```python
from build123d import *

# Parameters (mm, degrees)
BOSS_EXTRUDE1_DEPTH = 52.5
RIB1_REACH          = 184.705
SKETCH3_WALL_W      = 451.226000884
SKETCH3_WALL_H      = 25
RIB2_REACH          = 184.705
SKETCH2_WALL_W      = 451.226000884
SKETCH2_WALL_H      = 25
CUT_EXTRUDE1_DEPTH  = 31


with BuildPart() as part:
    # Sketch1 → Boss-Extrude1 (new, symmetric)
    with BuildSketch(Plane(origin=(0, 0, 0), x_dir=(0, 0, -1), z_dir=(1, 0, 0))):
        with BuildLine():
            Line((45, 0), (105, 0))
            Line((105, 0), (105, 60))
            Line((105, 60), (80, 60))
            Line((80, 60), (80, 140))
            Line((80, 140), (20, 140))
            Line((20, 140), (20, 126.52173913))
            Line((20, 126.52173913), (45, 126.52173913))
            Line((45, 126.52173913), (45, 90))
            Line((45, 90), (-45, 90))
            Line((-45, 90), (-45, 126.52173913))
            Line((-45, 126.52173913), (-20, 126.52173913))
            Line((-20, 126.52173913), (-20, 140))
            Line((-20, 140), (-80, 140))
            Line((-80, 140), (-80, 60))
            Line((-80, 60), (-105, 60))
            Line((-105, 60), (-105, 0))
            Line((-105, 0), (-45, 0))
            ThreePointArc((-45, 0), (0, 45), (45, 0))
        make_face()
    extrude(amount=BOSS_EXTRUDE1_DEPTH, both=True)

    # Sketch3 wall → Rib1 (add, up to next)
    with BuildSketch(Plane(origin=(0, 100, 92.5), x_dir=(0, -0.954479978035, 0.298274993136), z_dir=(0, -0.298274993136, -0.954479978035)), mode=Mode.PRIVATE) as rib1_sk1:
        Rectangle(SKETCH3_WALL_W, SKETCH3_WALL_H)
    rib1_tool1 = extrude(rib1_sk1.sketch, amount=RIB1_REACH, mode=Mode.PRIVATE) - part.part
    add(rib1_tool1.solids().sort_by_distance((0, 100, 92.5))[0])

    # Sketch2 wall → Rib2 (add, up to next)
    with BuildSketch(Plane(origin=(0, 100, -92.5), x_dir=(0, -0.954479978035, -0.298274993136), z_dir=(0, 0.298274993136, -0.954479978035)), mode=Mode.PRIVATE) as rib2_sk1:
        Rectangle(SKETCH2_WALL_W, SKETCH2_WALL_H)
    rib2_tool1 = extrude(rib2_sk1.sketch, amount=-RIB2_REACH, mode=Mode.PRIVATE) - part.part
    add(rib2_tool1.solids().sort_by_distance((0, 100, -92.5))[0])

    # Sketch5 → Cut-Extrude1 (cut)
    with BuildSketch(Plane(origin=(0, 140, 0), x_dir=(1, 0, 0), z_dir=(0, 1, 0))):
        with BuildLine():
            Line((31.721443851, -20), (-31.721443851, -20))
            ThreePointArc((-31.721443851, -20), (0, -37.5), (31.721443851, -20))
        make_face()
        with BuildLine():
            Line((31.721443851, 20), (-31.721443851, 20))
            ThreePointArc((-31.721443851, 20), (0, 37.5), (31.721443851, 20))
        make_face()
    extrude(amount=-CUT_EXTRUDE1_DEPTH, mode=Mode.SUBTRACT)


solid = part.part
```
The listing builds one solid part. Answer for the finished solid, in the listing's coordinates (mm). A direction names the side the tool comes from. Give positions to 0.01 mm unless a question says otherwise; leave off trailing zeros. Order: outer loops, then holes, each group sorted by start corner. A loop starts at its lowest first (then second) coordinate and runs counter-clockwise, first axis right, second up.
1) Determine the mould class of faces 4 (the face through (12.5, 90, 89)), 5 (the face through (-0.529, 133.355, 37.496)), 6 (the face through (33, 99, -80)) for opening direction X: pulls with the +X half, pulls with the -X half, needs draft (parallel to the pull), parting line crosses it, or undercut.
Reported:
face 4: pulls with the +X half
face 5: undercut
face 6: needs draft
2) Find section B-B on y = 106.5. Write down the section's boundary in (x, z).
Reported:
outline: (-52.5, -80) - (-12.5, -80) - (-12.5, -90.47) - (12.5, -90.47) - (12.5, -80) - (52.5, -80) - (52.5, -45) - (-52.5, -45) - close; (-52.5, 45) - (52.5, 45) - (52.5, 80) - (12.5, 80) - (12.5, 90.47) - (-12.5, 90.47) - (-12.5, 80) - (-52.5, 80) - close
3) Find section A-A on z = 41.5. Write down the section's boundary in (x, y), then the cut area to 3 significant figures.
Reported:
outline: (-52.5, 17.4) - (52.5, 17.4) - (52.5, 90) - (-52.5, 90) - close; (-52.5, 126.52) - (52.5, 126.52) - (52.5, 140) - (-52.5, 140) - close
area: 9,040 mm2
4) For faces 1 (the face through (-32, 99, -80)), 2 (the face through (-42, 133, -20)), 3 (the face through (33, 60, 92)), determine the directions among +Z, -Z, +X, -X, +Y, -Y from which every point of the face is accessible in a straight line to the end or side of a thin tool.
Reported:
face 1: -Z, -X, +Y
face 2: +X, -X, +Y
face 3: +Z, +X, +Y
5) Find section D-D on y = 84.5. Write down the section's boundary in (x, z), then the cut area to 3 significant figures.
Reported:
outline: (-52.5, -80) - (-12.5, -80) - (-12.5, -97.34) - (12.5, -97.34) - (12.5, -80) - (52.5, -80) - (52.5, 80) - (12.5, 80) - (12.5, 97.34) - (-12.5, 97.34) - (-12.5, 80) - (-52.5, 80) - close
area: 17,700 mm2
6) Given P1, Ø12, axis at x = -33, y = 99, coming from the +Z side; P2, Ø12.5, axis at x = 31, z = 90.5, coming from the +Y side; P3, Ø7.5, axis at x = 5.5, z = -36.5, coming from the -Y side; P4, Ø20, axis at y = 116.5, z = -98.5, coming from the +X side, each flat-ended and moving along its own axis, determine where each tip first touches the part or whether it passes through.
Reported:
P1: stops at z = 80
P2: stops at y = 60
P3: stops at y = 20.12
P4: passes through
7) Find section C-C on x = 22.5. Write down the section's boundary in (y, z), then the cut area to 3 significant figures.
Reported:
outline: (0, -105) - (60, -105) - (60, -80) - (140, -80) - (140, -30) - (126.52, -30) - (126.52, -45) - (90, -45) - (90, 45) - (126.52, 45) - (126.52, 30) - (140, 30) - (140, 80) - (60, 80) - (60, 105) - (0, 105) - (0, 45) arc R45 cw to (0, -45) - close
area: 18,100 mm2
8) Consider line 1 along Z through (x, y) = (-44.5, 123); line 2 along Y through (x, z) = (-25, 94); line 3 along X through (y, z) = (83.5, -94.5). Determine where each line is inside the solid, lowest interval first.
Reported:
line 1: z = -80 to -45, 45 to 80
line 2: y = 0 to 60
line 3: x = -12.5 to 12.5
